Read the model definition and answer for the solid it produces. Units are mm, in the model's axes. Face numbers are marked on the shaded views. A direction names the side the tool comes from. Coordinates: 2 decimals unless noted, no trailing zeros. Loops run counter-clockwise (first coordinate to the right, second up) from the corner with the lowest first, then second, coordinate; pieces in that order, holes last. Notation, with made-up numbers: (-1.75, -32.5) - (53.25, -32.5) arc R32 ccw to (53.25, 6.5) - close; hole circle Ø6 at (49.5, 48). An arc over 180 degrees is marked (long way). Use one line per item in the form item = value.
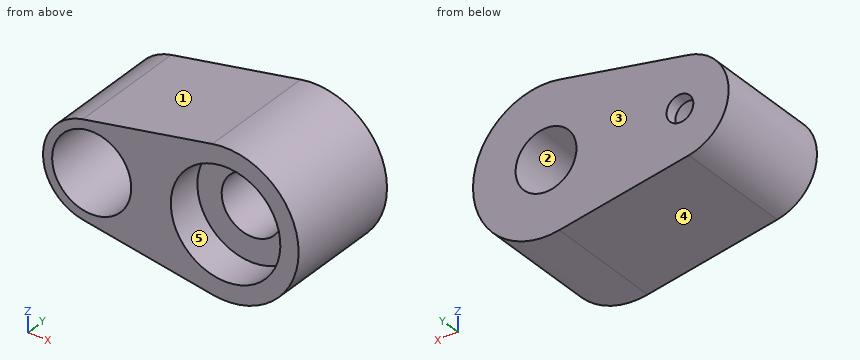
from build123d import *

# Parameters (mm, degrees)
SKETCH_1_R          = 1.5
SKETCH_1_R_2        = 1.1
EXTRUDE_1_DEPTH     = 6.5
EXTRUDE_START       = 1
SKETCH_2_R          = 4
SKETCH_2_R_2        = 1.1
EXTRUDE_2_DEPTH     = 1
EXTRUDE_START_2     = 9
SKETCH_3_R          = 4
SKETCH_3_R_2        = 3.25
EXTRUDE_3_DEPTH     = 9
EXTRUDE_START_3     = -10
SKETCH_4_R          = 2.5
EXTRUDE_4_DEPTH     = 10
SKETCH_5_R          = 4.5
CUT_EXTRUDE_1_DEPTH = 3
CUT_EXTRUDE_START   = -6.5
SKETCH_7_R          = 1.5
CUT_EXTRUDE_2_DEPTH = 6.5


with BuildPart() as part:
    # Эскиз1 → Бобышка-Вытянуть1 (new body)
    with BuildSketch(Plane(origin=(0, 0, 0), x_dir=(1, 0, 0), z_dir=(0, 1, 0))):
        with Locations(Location((0, 0, 0), (0, 0, 90))):
            Circle(SKETCH_1_R)
        with Locations(Location((0, 0, 0), (0, 0, 90))):
            Circle(SKETCH_1_R_2, mode=Mode.SUBTRACT)
    extrude(amount=EXTRUDE_1_DEPTH)

    # Эскиз2 → Бобышка-Вытянуть2 (add)
    with BuildSketch(Plane.XZ.offset(EXTRUDE_START)):
        with Locations(Location((0, 0, 0), (0, 0, 270))):
            Circle(SKETCH_2_R)
        with Locations(Location((0, 0, 0), (0, 0, 270))):
            Circle(SKETCH_2_R_2, mode=Mode.SUBTRACT)
    extrude(amount=-EXTRUDE_2_DEPTH)

    # Эскиз3 → Бобышка-Вытянуть3 (add)
    with BuildSketch(Plane.XZ.offset(1).offset(EXTRUDE_START_2)):
        with Locations(Location((0, 0, 0), (0, 0, 270))):
            Circle(SKETCH_3_R)
        with Locations(Location((0, 0, 0), (0, 0, 270))):
            Circle(SKETCH_3_R_2, mode=Mode.SUBTRACT)
    extrude(amount=-EXTRUDE_3_DEPTH)

    # Эскиз4 → Бобышка-Вытянуть4 (add)
    with BuildSketch(Plane(origin=(0, 0, 0), x_dir=(1, 0, 0), z_dir=(0, 1, 0)).offset(EXTRUDE_START_3)):
        with BuildLine():
            ThreePointArc((-0.727272727, 3.933328664), (4, 0), (-0.727272727, -3.933328664))
            Line((-0.727272727, -3.933328664), (9.909090909, -5.899992996))
            ThreePointArc((9.909090909, -5.899992996), (17, 0), (9.909090909, 5.899992996))
            Line((9.909090909, 5.899992996), (-0.727272727, 3.933328664))
        make_face()
        with Locations(Location((11, 0, 0), (0, 0, 270))):
            Circle(SKETCH_4_R, mode=Mode.SUBTRACT)
    extrude(amount=EXTRUDE_4_DEPTH)

    # Эскиз5 → Вырез-Вытянуть1 (cut)
    with BuildSketch(Plane.XZ.offset(10)):
        with Locations(Location((11, 0, 0), (0, 0, 270))):
            Circle(SKETCH_5_R)
    extrude(amount=-CUT_EXTRUDE_1_DEPTH, mode=Mode.SUBTRACT)

    # Эскиз7 → Вырез-Вытянуть2 (cut)
    with BuildSketch(Plane(origin=(0, 6.5, 0), x_dir=(1, 0, 0), z_dir=(0, 1, 0)).offset(CUT_EXTRUDE_START)):
        Circle(SKETCH_7_R)
    extrude(amount=CUT_EXTRUDE_2_DEPTH, mode=Mode.SUBTRACT)


solid = part.part
Item 1: The part is cut by section C-C on y = -7.25. Give the vertices of the cut face in (x, z).
Results below:
outline = (-0.73, -3.93) - (9.91, -5.9) arc R6 ccw (long way) to (9.91, 5.9) - (-0.73, 3.93) arc R4 ccw to start; hole circle Ø6.5 at (0, 0); hole circle Ø9 at (11, 0)
Item 2: For a pull along X with two mould halves and no side action, classify the marked faces 1, 2 and 3 as +X half, -X half, draft (parallel to the pull), parting line (faces both ways), or undercut.
Results below:
face_1 = -X half
face_2 = undercut
face_3 = draft
Item 3: The part is cut by section B-B on z = 0. Give the vertices of the cut face in (x, y).
Results below:
outline = (-4, -10) - (-3.25, -10) - (-3.25, -1) - (-1.1, -1) - (-1.1, 0) - (-4, 0) - close; (1.1, -1) - (3.25, -1) - (3.25, -10) - (6.5, -10) - (6.5, -7) - (8.5, -7) - (8.5, 0) - (1.1, 0) - close; (13.5, -7) - (15.5, -7) - (15.5, -10) - (17, -10) - (17, 0) - (13.5, 0) - close
Item 4: The part is cut by section A-A on x = 11. Give the vertices of the cut face in (y, z), plus the area to 3 significant figures.
Results below:
outline = (-10, -6) - (0, -6) - (0, -2.5) - (-7, -2.5) - (-7, -4.5) - (-10, -4.5) - close; (-10, 4.5) - (-7, 4.5) - (-7, 2.5) - (0, 2.5) - (0, 6) - (-10, 6) - close
area = 58.0 mm²
Item 5: Each of these flat-tipped pins is pushed along its axis until it touches: P1, Ø2, axis at x = -1, z = -1.5, coming from the -Y side; P2, Ø1, axis at y = -7.5, z = 4.5, coming from the +X side; P3, Ø4.5, axis at x = 11, z = 0, coming from the -Y side; P4, Ø5.5, axis at x = 11, z = 0, coming from the -Y side. Where does it stop, or does it pass through?
Results below:
P1 = -1
P2 = 15.47
P3 = through
P4 = -7
Item 6: The part is cut by section D-D on z = 4.25. Give the vertices of the cut face in (x, y), plus the area to 3 significant figures.
Results below:
outline = (0.99, -10) - (9.52, -10) - (9.52, -7) - (12.48, -7) - (12.48, -10) - (15.24, -10) - (15.24, 0) - (0.99, 0) - close
area = 134 mm²
Item 7: Which of the six approach directions +Z, -Z, +X, -X, +Y, -Y give full straight-line access (tool end or side, diameter ignored) to the marked faces 4 and 5?
Results below:
face_4 = -Z, -X, +Y, -Y
face_5 = -Y
Item 8: Find the intervals of material crossed by L1, parallel to X at y = -8.95, z = 0; L2, parallel to Z at x = 11, y = -4.5; L3, parallel to X at y = -1.5, z = -0.5, in increasing order.
Results below:
L1 = -4 to -3.25, 3.25 to 6.5, 15.5 to 17
L2 = -6 to -2.5, 2.5 to 6
L3 = -3.97 to -3.21, 3.21 to 8.55, 13.45 to 16.98
